Answer from the drawing. Dimensions are ordinates in mm from the lowest x, y and z of the part. A direction names the side the tool comes from. Coordinates: 2 decimals unless noted, no trailing zeros. Write each loop counter-clockwise with the first axis right and the second up, starting at its lowest first coordinate (ties: lowest second). Pieces come first, ordered by that corner, then holes. Notation, with made-up numbers: (4.5, 45.5) -> (37.5, 45.5) arc R21 cw to (37.5, 79.5) -> close; hole circle Ø8 at (36.25, 48). An arc over 180 degrees is marked (long way). Answer as a JSON object with one key per item and string values. Group by question number.
(1) Which of the six approach directions +Z, -Z, +X, -X, +Y, -Y give full straight-line access (tool end or side, diameter ignored) to the marked faces 1 and 2?
(2) Find section A-A (z = 10). Give the vertices of the cut face in (x, y), then the cut area to 3 significant figures.
(3) Find section C-C (y = 3.9). Give the vertices of the cut face in (x, z).
(4) Find section B-B (x = 10). Give the vertices of the cut face in (y, z).
(5) Straight lines are drawn through the part: L1, parallel to X at y = 0.8, z = 10; L2, parallel to Y at x = 12.75, z = 7.75; L3, parallel to X at y = 3.85, z = 11.75 (1 decimal). For each, find the intervals that lie inside material, in ascending order.
(6) Find section D-D (y = 0.8). Give the vertices of the cut face in (x, z).
(7) For a pull along Z with two mould halves and no side action, classify the marked faces 3, 4 and 5 as +Z half, -Z half, draft (parallel to the pull), parting line (faces both ways), or undercut.
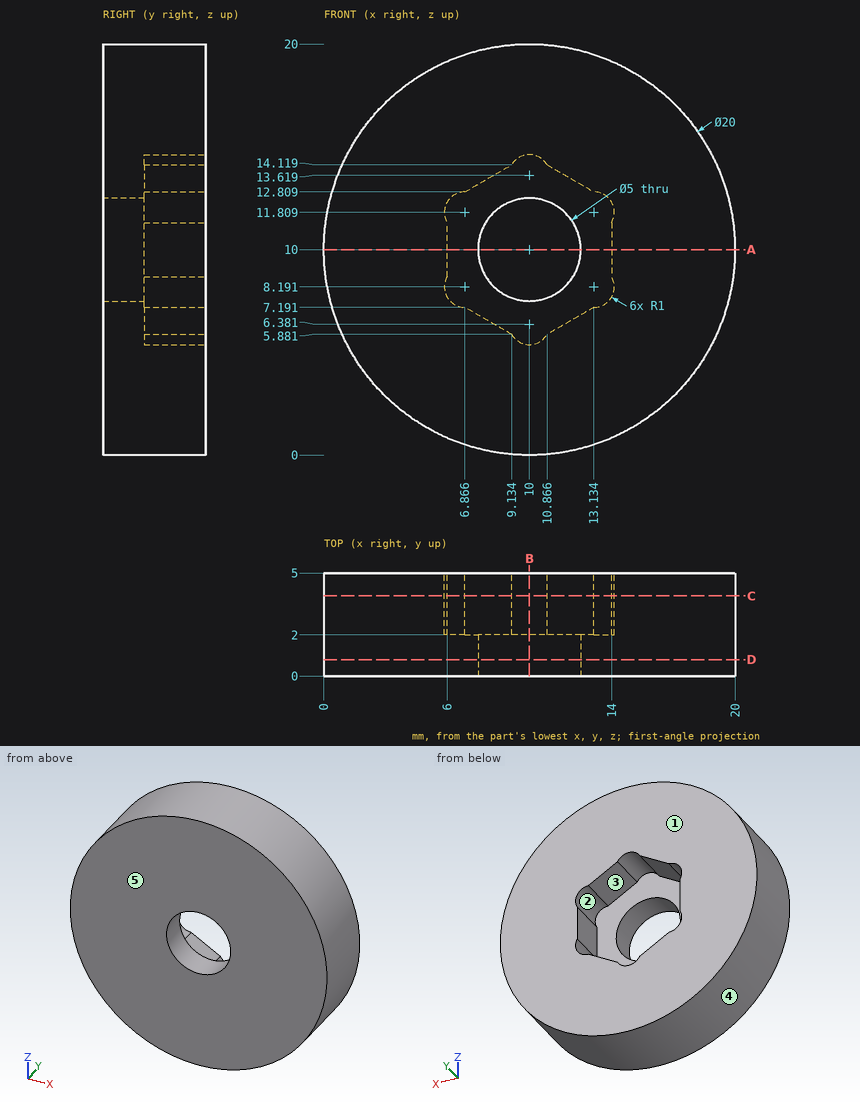
Results below:
{
 "1": {"face 1": "+Z, -Z, +X, -X, +Y", "face 2": "+Y"},
 "2": {"outline": "(0, 0) -> (7.5, 0) -> (7.5, 2) -> (6, 2) -> (6, 5) -> (0, 5) -> close; (12.5, 0) -> (20, 0) -> (20, 5) -> (14, 5) -> (14, 2) -> (12.5, 2) -> close", "area": "66.0 mm2"},
 "3": {"outline": "circle Ø20 at (10, 10); hole (6, 8.69) arc R1 ccw to (6.87, 7.19) -> (9.13, 5.88) arc R1 ccw to (10.87, 5.88) -> (13.13, 7.19) arc R1 ccw to (14, 8.69) -> (14, 11.31) arc R1 ccw to (13.13, 12.81) -> (10.87, 14.12) arc R1 ccw to (9.13, 14.12) -> (6.87, 12.81) arc R1 ccw to (6, 11.31) -> close"},
 "4": {"outline": "(0, 0) -> (5, 0) -> (5, 5.38) -> (2, 5.38) -> (2, 7.5) -> (0, 7.5) -> close; (0, 12.5) -> (2, 12.5) -> (2, 14.62) -> (5, 14.62) -> (5, 20) -> (0, 20) -> close"},
 "5": {"L1": "x = 0 to 7.5, 12.5 to 20", "L2": "y = 0 to 2", "L3": "x = 0.2 to 5.9, 14.1 to 19.8"},
 "6": {"outline": "circle Ø20 at (10, 10); hole circle Ø5 at (10, 10)"},
 "7": {"face 3": "undercut", "face 4": "parting line", "face 5": "draft"}
}
